The drawing under review shows one solid part. Ordinate dimensions are in mm from its lowest x, y, z. Give positions to 0.01 mm unless a question says otherwise; leave off trailing zeros. Order: outer loops, then holes, each group sorted by start corner. A loop starts at its lowest first (then second) coordinate and runs counter-clockwise, first axis right, second up. Notation, with made-up numbers: (-7, 86) -> (27, 86) arc R19 ccw to (27, 99) -> close; hole circle Ø10 at (24, 15). An arc over 180 degrees is marked (long way). Return JSON: item names as keys, results as strings. Group by question number.
1) To check wall thickness, follow line 1 along X through (y, z) = (2.25, 39); line 2 along Z through (x, y) = (17, 1.75) (1 decimal); line 3 along Z through (x, y) = (8.75, 7.25) (1 decimal). State the ranges of each line that lie inside material, in increasing order.
2) Add section C-C (y = 6.25). Give the boundary of the cut face in (x, z).
3) Add section B-B (z = 34). Give the boundary of the cut face in (x, y).
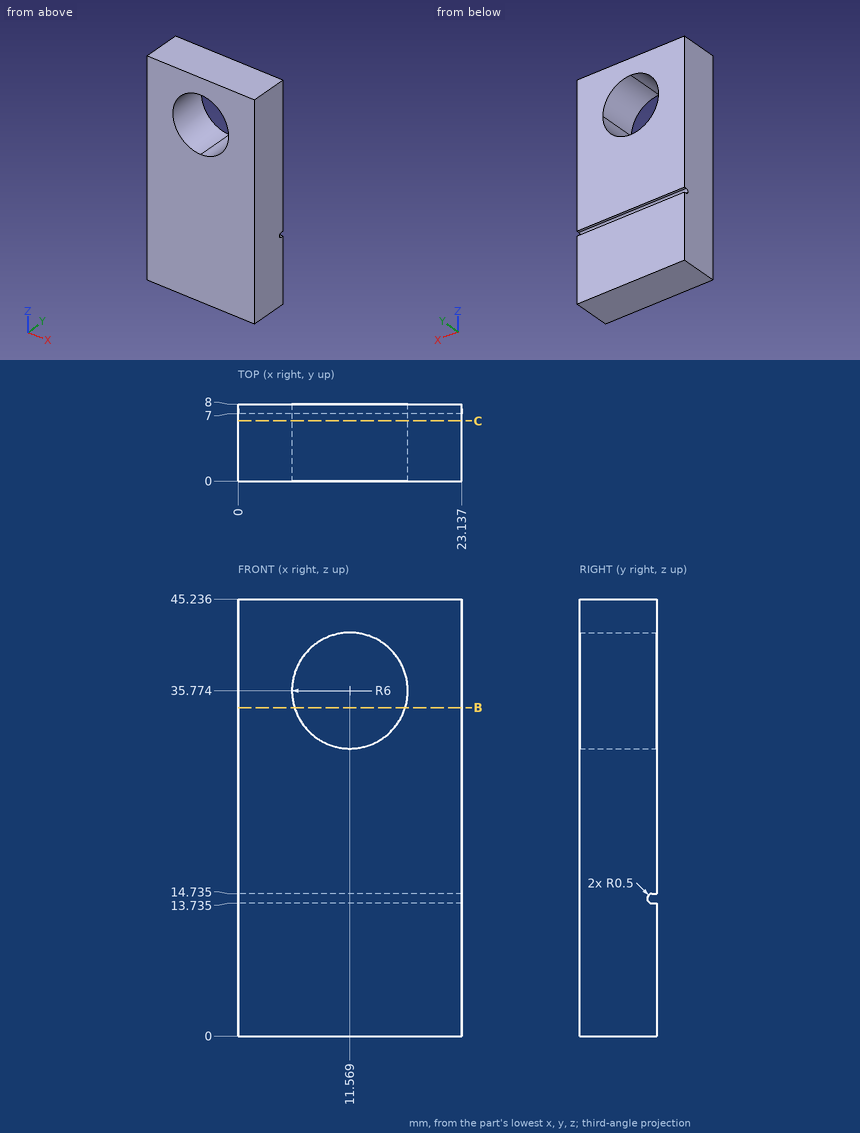
Evaluation:
{
 "1": {"line 1": "0 to 6.51, 16.63 to 23.14", "line 2": "0 to 33.2, 38.3 to 45.2", "line 3": "0 to 13.8, 14.7 to 30.5, 41.1 to 45.2"},
 "2": {"outline": "(0, 0) -> (23.14, 0) -> (23.14, 45.24) -> (0, 45.24) -> close; hole circle Ø12 at (11.57, 35.77)"},
 "3": {"outline": "(0, 0) -> (5.84, 0) -> (5.84, 8) -> (0, 8) -> close; (17.3, 0) -> (23.14, 0) -> (23.14, 8) -> (17.3, 8) -> close"}
}
